Study the drawing (mm; zero at the part's minimum x, y, z) and answer. A direction names the side the tool comes from. Round coordinates to 2 decimals unless told otherwise and drop trailing zeros. Order: outer loops, then holes, each group sorted by start corner. A loop starts at its lowest first (then second) coordinate and runs counter-clockwise, first axis right, second up. Notation, with made-up numbers: (33, -7.75) - (74, -7.75) arc R12 cw to (74, 0.25) - close; hole circle Ø11 at (-21.5, -4.75). An arc over 180 degrees is marked (long way). Put each result on its own line as item: value. Start each with the question number.
Q1. Find the intervals of material crossed by line 1 along Z through (x, y) = (18, 17); line 2 along Z through (x, y) = (32.5, 23.25); line 3 along X through (y, z) = (21.25, 24), in increasing order. Write a range as from..to.
Q2. Section B-B on z = 14 is taken. Give the vertices of the cut face in (x, y), then the cut area to 3 significant figures.
Q3. Section C-C on z = 23 is taken. Give the vertices of the cut face in (x, y), then the cut area to 3 significant figures.
Q4. Section A-A on y = 23 is taken. Give the vertices of the cut face in (x, z).
Q5. Which of the six approach directions +Z, -Z, +X, -X, +Y, -Y give full straight-line access (tool end or side, diameter ignored) to the marked faces 1, 2 and 3?
Q6. Each of these flat-tipped pins is pushed along its axis until it touches: pin 1 Ø12 at (y, z) = (6, 17.5) entering from +X; pin 2 Ø8 at (x, y) = (21.5, 12.5) entering from +Z; pin 3 Ø6.5 at (x, z) = (27.5, 12) entering from -Y. Where does it stop, or does it pass through?
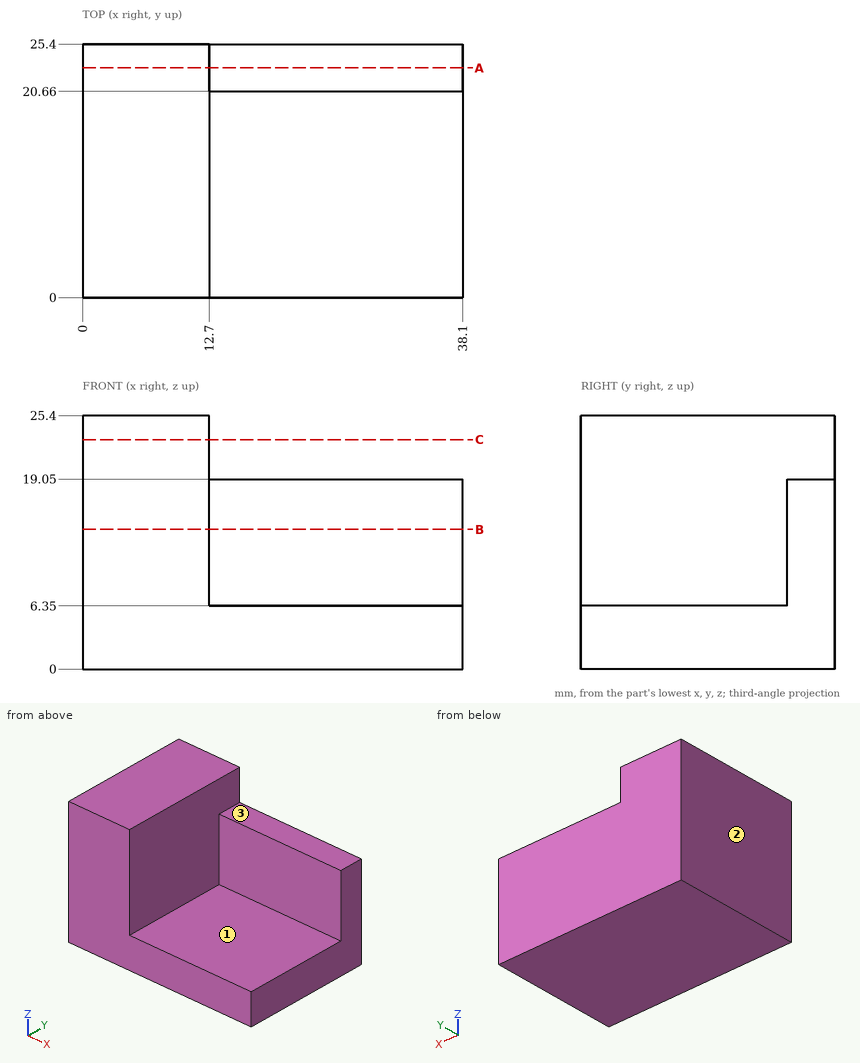
Findings:
1. line 1: 0..6.35
1. line 2: 0..19.05
1. line 3: 0..12.7
2. outline: (0, 0) - (12.7, 0) - (12.7, 20.66) - (38.1, 20.66) - (38.1, 25.4) - (0, 25.4) - close
2. area: 443 mm2
3. outline: (0, 0) - (12.7, 0) - (12.7, 25.4) - (0, 25.4) - close
3. area: 323 mm2
4. outline: (0, 0) - (38.1, 0) - (38.1, 19.05) - (12.7, 19.05) - (12.7, 25.4) - (0, 25.4) - close
5. face 1: +Z, +X, -Y
5. face 2: +Z, -Z, -X, +Y, -Y
5. face 3: +Z, +X, +Y, -Y
6. pin 1: x = 12.7
6. pin 2: z = 6.35
6. pin 3: y = 20.66
